Input: dimensioned drawing with shaded views. Units: mm. Origin: part minimum x, y, z. Coordinates: 2 decimals unless noted, no trailing zeros. Order: outer loops, then holes, each group sorted by start corner. A loop starts at its lowest first (then second) coordinate and runs counter-clockwise, first axis right, second up.
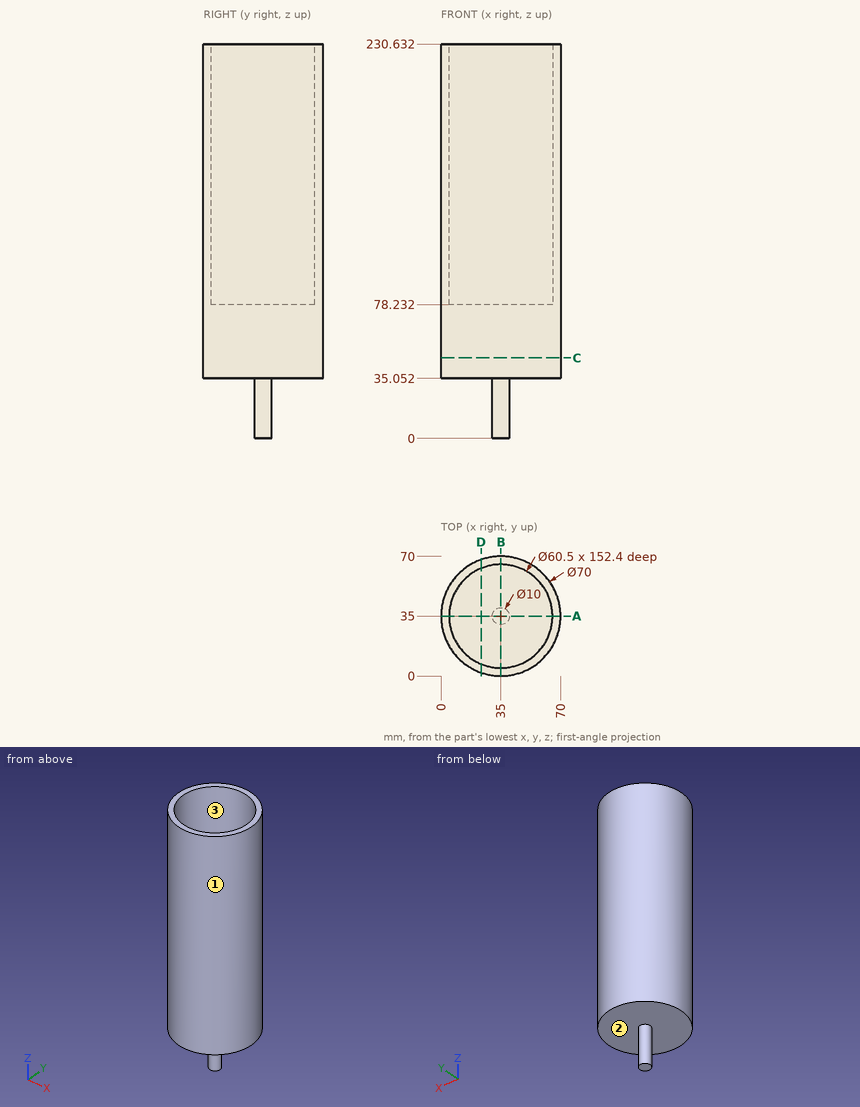
1. Section query A-A on y = 35. Return loops of the section in (x, z).
Findings:
outline: (0, 35.05) - (30, 35.05) - (30, 0) - (40, 0) - (40, 35.05) - (70, 35.05) - (70, 230.63) - (65.25, 230.63) - (65.25, 78.23) - (4.75, 78.23) - (4.75, 230.63) - (0, 230.63) - close
2. Section query C-C on z = 47. Return loops of the section in (x, y), plus the area to 3 significant figures.
Findings:
outline: circle Ø70 at (35, 35)
area: 3,850 mm2
3. Draft query along Y for the marked faces 1, 2 and 3. Return one class per face: released by +Y, released by -Y, zero draft, split by the parting line, or undercut.
Findings:
face 1: split by the parting line
face 2: zero draft
face 3: undercut
4. Pin query (flat end, axial travel): P1, Ø3, axis at x = 44.5, y = 16, coming from the +Z side; P2, Ø6, axis at x = 12, y = 46.5, coming from the -Z side; P3, Ø1, axis at y = 54, z = 154, coming from the -X side. Return the tip coordinate at first contact, or that it passes through.
Findings:
P1: stops at z = 78.23
P2: stops at z = 35.05
P3: stops at x = 5.29
5. Section query D-D on x = 23.5. Return loops of the section in (y, z).
Findings:
outline: (1.94, 35.05) - (68.06, 35.05) - (68.06, 230.63) - (62.98, 230.63) - (62.98, 78.23) - (7.02, 78.23) - (7.02, 230.63) - (1.94, 230.63) - close
6. Ray query, line 1 (Y direction, x = 35, z = 187); line 2 (Z direction, x = 8, y = 45.5); line 3 (Z direction, x = 32, y = 38.5). Return the intervals inside material, ascending.
Findings:
line 1: y = 0 to 4.75, 65.25 to 70
line 2: z = 35.05 to 78.23
line 3: z = 0 to 78.23
